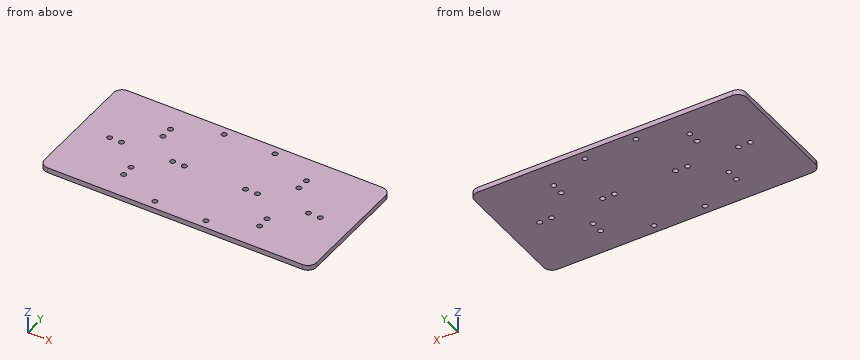
```python
from build123d import *

# Parameters (mm, degrees)
SKETCH_1_W          = 160
SKETCH_1_H          = 75
EXTRUDE_1_DEPTH     = 3
SKETCH_4_R          = 1.5
CUT_EXTRUDE_1_DEPTH = 3
SKETCH_5_R          = 1.5
CUT_EXTRUDE_2_DEPTH = 3
SKETCH_6_R          = 1.5
CUT_EXTRUDE_3_DEPTH = 3
FILLET_1_R          = 5
FILLET_2_R          = 5
FILLET_3_R          = 5
FILLET_4_R          = 5


with BuildPart() as part:
    # 草图1 → 凸台-拉伸1 (new body)
    with BuildSketch(Plane.XY):
        with Locations((80, -37.5)):
            Rectangle(SKETCH_1_W, SKETCH_1_H)
    extrude(amount=EXTRUDE_1_DEPTH)

    # 草图4 → 切除-拉伸1 (cut)
    with BuildSketch(Plane.XY.offset(3)):
        with Locations((40, -15.5)):
            Circle(SKETCH_4_R)
        with Locations((18, -37.5)):
            Circle(SKETCH_4_R)
        with Locations((62, -37.5)):
            Circle(SKETCH_4_R)
        with Locations((40, -59.5)):
            Circle(SKETCH_4_R)
        with Locations((40, -22.5)):
            Circle(SKETCH_4_R)
        with Locations((25, -37.5)):
            Circle(SKETCH_4_R)
        with Locations((55, -37.5)):
            Circle(SKETCH_4_R)
        with Locations((40, -52.5)):
            Circle(SKETCH_4_R)
    extrude(amount=-CUT_EXTRUDE_1_DEPTH, mode=Mode.SUBTRACT)

    # 草图5 → 切除-拉伸2 (cut)
    with BuildSketch(Plane.XY.offset(3)):
        with Locations((120, -15.5)):
            Circle(SKETCH_5_R)
        with Locations((98, -37.5)):
            Circle(SKETCH_5_R)
        with Locations((120, -59.5)):
            Circle(SKETCH_5_R)
        with Locations((142, -37.5)):
            Circle(SKETCH_5_R)
        with Locations((120, -22.5)):
            Circle(SKETCH_5_R)
        with Locations((105, -37.5)):
            Circle(SKETCH_5_R)
        with Locations((120, -52.5)):
            Circle(SKETCH_5_R)
        with Locations((135, -37.5)):
            Circle(SKETCH_5_R)
    extrude(amount=-CUT_EXTRUDE_2_DEPTH, mode=Mode.SUBTRACT)

    # 草图6 → 切除-拉伸3 (cut)
    with BuildSketch(Plane.XY.offset(3)):
        with Locations((65, -5)):
            Circle(SKETCH_6_R)
        with Locations((95, -5)):
            Circle(SKETCH_6_R)
        with Locations((65, -70)):
            Circle(SKETCH_6_R)
        with Locations((95, -70)):
            Circle(SKETCH_6_R)
    extrude(amount=-CUT_EXTRUDE_3_DEPTH, mode=Mode.SUBTRACT)

    # 圆角1
    fillet_1_edges = [part.edges().sort_by_distance(p)[0] for p in [
        (160, 0, 1.5),
    ]]
    fillet(fillet_1_edges, radius=FILLET_1_R)

    # 圆角2
    fillet_2_edges = [part.edges().sort_by_distance(p)[0] for p in [
        (0, 0, 1.5),
    ]]
    fillet(fillet_2_edges, radius=FILLET_2_R)

    # 圆角3
    fillet_3_edges = [part.edges().sort_by_distance(p)[0] for p in [
        (0, -75, 1.5),
    ]]
    fillet(fillet_3_edges, radius=FILLET_3_R)

    # 圆角4
    fillet_4_edges = [part.edges().sort_by_distance(p)[0] for p in [
        (160, -75, 1.5),
    ]]
    fillet(fillet_4_edges, radius=FILLET_4_R)


solid = part.part
```
Here's how the part is built. I have some questions about the finished solid (model axes, mm). Coordinates: 2 decimals unless noted, no trailing zeros. Write each loop counter-clockwise with the first axis right and the second up, starting at its lowest first coordinate (ties: lowest second). Pieces come first, ordered by that corner, then holes. Notation, with made-up numbers: (-6, 73) - (40, 73) arc R32 cw to (40, 101) - close; hole circle Ø6 at (-23.5, 32.25). An arc over 180 degrees is marked (long way). One line per item, written item: value.
1) Suppose I cut it at B-B on x = 142. Write out the boundary of the cut face in (y, z), and give its area (3 significant figures).
Model answer:
outline: (-75, 0) - (-39, 0) - (-39, 3) - (-75, 3) - close; (-36, 0) - (0, 0) - (0, 3) - (-36, 3) - close
area: 216 mm²
2) Suppose I cut it at A-A on y = -15.5. Write out the boundary of the cut face in (x, z).
Model answer:
outline: (0, 0) - (38.5, 0) - (38.5, 3) - (0, 3) - close; (41.5, 0) - (118.5, 0) - (118.5, 3) - (41.5, 3) - close; (121.5, 0) - (160, 0) - (160, 3) - (121.5, 3) - close
3) Suppose I cut it at C-C on x = 40. Write out the boundary of the cut face in (y, z).
Model answer:
outline: (-75, 0) - (-61, 0) - (-61, 3) - (-75, 3) - close; (-58, 0) - (-54, 0) - (-54, 3) - (-58, 3) - close; (-51, 0) - (-24, 0) - (-24, 3) - (-51, 3) - close; (-21, 0) - (-17, 0) - (-17, 3) - (-21, 3) - close; (-14, 0) - (0, 0) - (0, 3) - (-14, 3) - close
4) I need wall thicknesses on line 1 along Y through (x, z) = (65, 1.9); line 2 along Y through (x, z) = (120, 2); line 3 along Y through (x, z) = (98, 0.9). Which ranges of each line are inside material? Lowest first, please.
Model answer:
line 1: y = -75 to -71.5, -68.5 to -6.5, -3.5 to 0
line 2: y = -75 to -61, -58 to -54, -51 to -24, -21 to -17, -14 to 0
line 3: y = -75 to -39, -36 to 0
5) I'm going to push a flat-ended pin straight in: P1, Ø2.5, axis at x = 120, y = -52.5, coming from the -Z side. Where does the tip first touch, or does it pass through?
Model answer:
P1: passes through
